Read the model definition and answer for the solid it produces. Units are mm, in the model's axes. Face numbers are marked on the shaded views. A direction names the side the tool comes from. Give positions to 0.01 mm unless a question says otherwise; leave off trailing zeros. Write each loop counter-clockwise with the first axis right and the second up, starting at its lowest first coordinate (ties: lowest second). Pieces come first, ordered by that corner, then holes.
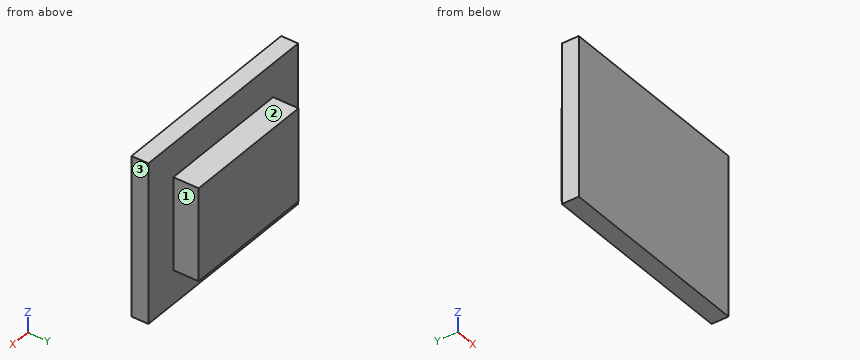
Autodesk Inventor part; units mm, degrees
ref_plane "YZ Plane" through (0, 0, 0) normal (1, 0, 0) x (0, 1, 0)
ref_plane "XZ Plane" through (0, 0, 0) normal (0, 1, 0) x (-1, 0, 0)
ref_plane "XY Plane" through (0, 0, 0) normal (0, 0, 1) x (1, 0, 0)
sketch "Sketch1" plane through (0, 0, 0) normal (0, 1, 0) x (-1, 0, 0)
  line L0 (0, 0) -> (-8, 0)
  line L1 (-8, 0) -> (-8, 6)
  line L2 (-8, 6) -> (0, 6)
  line L3 (0, 6) -> (0, 0)
  dimension "d0" = 8
  dimension "d1" = 6
extrude "Extrusion1" add sketch "Sketch1" along normal blind 1.5
sketch "Sketch2" plane through (0, 0, 0) normal (0, -1, 0) x (1, 0, 0)
  line L0 (8, 0) -> (0, 0)
  line L1 (8, 0) -> (0, 0)
  line L2 (8, 6) -> (8, 0)
  line L3 (0, 6) -> (8, 6)
  line L4 (8, 6) -> (8, 0)
  line L5 (0, 5.5) -> (8, 5.5)
  line L6 (0, 5.5) -> (0, 6)
  line L7 (0, 6) -> (8, 6)
  line L8 (8, 6) -> (8, 5.5)
  line L9 (8, 6) -> (0, 6)
  dimension "d4" = 5.5
extrude "Extrusion2" cut sketch "Sketch2" against normal blind 10
sketch "Sketch3" plane through (0, 0, 0) normal (0, -1, 0) x (1, 0, 0)
  point P0 (0, 0)
sketch "Sketch4" plane through (0, 0, 0) normal (0, -1, 0) x (1, 0, 0)
  line L0 (8, 0) -> (0, 0)
  line L1 (0, -2) -> (10, -2)
  line L2 (10, -2) -> (10, 7.5)
  line L3 (10, 7.5) -> (-2, 7.5)
  line L4 (-2, 7.5) -> (-2, -2)
  line L5 (-2, -2) -> (0, -2)
  dimension "d7" = 2
  dimension "d8" = 10
  dimension "d9" = 9.5
  dimension "d10" = 12
extrude "Extrusion3" add sketch "Sketch4" along normal blind 1
properties part number "Button"
Item 1: Section C-C (y = 0.5) is taken. Write down the section's boundary in (x, z), and give its area (3 significant figures).
Result set:
outline: (0, 0) - (8, 0) - (8, 5.5) - (0, 5.5) - close
area: 44.0 mm2
Item 2: Find the intervals of material crossed by line 1 along Z through (x, y) = (6.5, 0.35); line 2 along Y through (x, z) = (7.75, 5.75); line 3 along X through (y, z) = (1.25, 4), in increasing order.
Result set:
line 1: z = 0 to 5.5
line 2: y = -1 to 0
line 3: x = 0 to 8
Item 3: Section B-B (x = 7.25) is taken. Write down the section's boundary in (y, z), and give its area (4 significant figures).
Result set:
outline: (-1, -2) - (0, -2) - (0, 0) - (1.5, 0) - (1.5, 5.5) - (0, 5.5) - (0, 7.5) - (-1, 7.5) - close
area: 17.75 mm2
Item 4: Section A-A (z = 0.5) is taken. Write down the section's boundary in (x, y), and give its area (3 significant figures).
Result set:
outline: (-2, -1) - (10, -1) - (10, 0) - (8, 0) - (8, 1.5) - (0, 1.5) - (0, 0) - (-2, 0) - close
area: 24.0 mm2
Item 5: Section D-D (z = 7) is taken. Write down the section's boundary in (x, y), and give its area (3 significant figures).
Result set:
outline: (-2, -1) - (10, -1) - (10, 0) - (-2, 0) - close
area: 12.0 mm2
Item 6: Which of the six approach directions +Z, -Z, +X, -X, +Y, -Y give full straight-line access (tool end or side, diameter ignored) to the marked faces 1, 2 and 3?
Result set:
face 1: +Z, -Z, +X, +Y
face 2: +Z, +X, -X, +Y
face 3: +Z, -Z, +X, +Y, -Y
